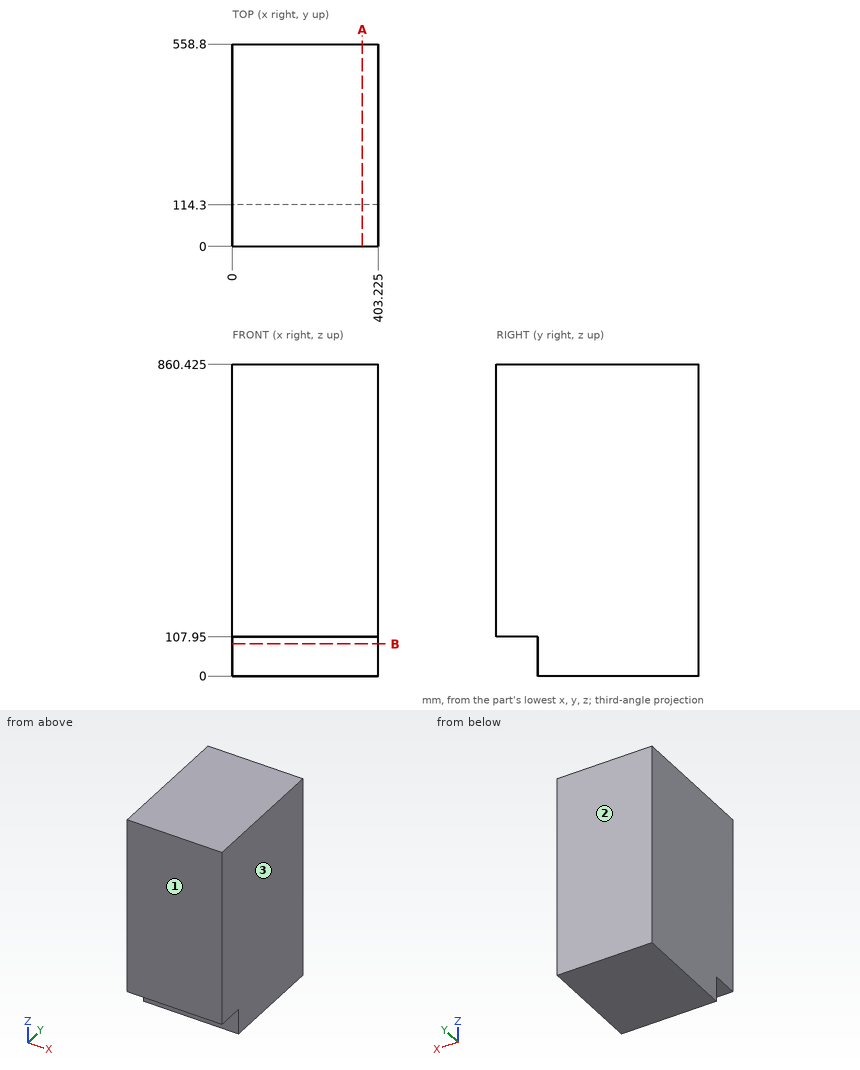
The drawing under review shows one solid part. Ordinate dimensions are in mm from its lowest x, y, z. Round coordinates to 2 decimals unless told otherwise and drop trailing zeros. Write each loop counter-clockwise with the first axis right and the second up, starting at its lowest first coordinate (ties: lowest second). Pieces come first, ordered by that corner, then holes. Notation, with made-up numbers: M -36.75,29 L -16.75,29 A9 cw -16.75,42 Z; hole C 86,39 d2. An arc over 180 degrees is marked long. One line per item, written item: value. Start each with the question number.
(1) The part is to be moulded in two halves that separate along Y. For the marked faces 1, 2 and 3, say which applies: released by +Y, released by -Y, zero draft, split by the parting line, or undercut.
(2) We need section A-A (x = 359.5). Give the boundary of the cut face in (y, z) (3 decimals), and give its area (3 significant figures).
(3) We need section B-B (z = 89). Give the boundary of the cut face in (x, y) (3 decimals).
(4) Wall thickness on line 1 (Z direction, x = 127, y = 110) (3 decimals): over which ranges is the line inside the solid? List them lowest first.
Result:
1. face 1: released by -Y
1. face 2: released by +Y
1. face 3: zero draft
2. outline: M 0,107.95 L 114.3,107.95 L 114.3,0 L 558.8,0 L 558.8,860.425 L 0,860.425 Z
2. area: 468,000 mm²
3. outline: M 0,114.3 L 403.225,114.3 L 403.225,558.8 L 0,558.8 Z
4. line 1: 107.95 to 860.425
